from build123d import *

# Parameters (mm, degrees)
F1_DEPTH = 25.4
F2_W     = 50.8
F2_H     = 317.5
F3_DEPTH = 38.1
F4_W     = 50.8
F4_H     = 76.2
F5_DEPTH = 660.4
F7_DEPTH = 25.4
F8_W     = 1196.34
F8_H     = 25.4
F9_DEPTH = 304.8


# Not quite as in the source:
# - a feature names something its author has since deleted; it is built from what else it names


with BuildPart() as f1:
    # F0 (on Top) → F1 (new body)
    with BuildSketch(Plane.XY):
        Polygon((-674.37, -342.9), (674.37, -342.9), (674.37, 342.9), (-674.37, 342.9), (-674.37, -114.3), align=None)
    extrude(amount=F1_DEPTH)

    # F2 (on face) → F3 (join)
    with BuildSketch(Plane.XY.offset(25.4)):
        with Locations((-623.57, 44.45)):
            Rectangle(F2_W, F2_H)
        with Locations((623.57, 44.45)):
            Rectangle(F2_W, F2_H)
    extrude(amount=F3_DEPTH)

    # F4 (on face) → F5 (join)
    with BuildSketch(Plane.XY.offset(25.4)):
        with Locations((-623.57, -152.4)):
            Rectangle(F4_W, F4_H)
        with Locations((623.57, -152.4)):
            Rectangle(F4_W, F4_H)
    extrude(amount=F5_DEPTH)

    # F6 (on face) → F7 (join)
    with BuildSketch(Plane.XY.offset(685.8)):
        with BuildLine():
            ThreePointArc((-623.6857005119, -267.7317205817), (-605.7251882698, -260.2922328238), (-598.2857005119, -242.3317205817))
            Line((-598.2857005119, -242.3317205817), (-598.2857005119, 214.8682794183))
            ThreePointArc((-598.2857005119, 214.8682794183), (-605.7251882698, 232.8287916605), (-623.6857005119, 240.2682794183))
            ThreePointArc((-623.6857005119, 240.2682794183), (-641.6462127541, 232.8287916605), (-649.0857005119, 214.8682794183))
            Line((-649.0857005119, 214.8682794183), (-649.0857005119, -242.3317205817))
            ThreePointArc((-649.0857005119, -242.3317205817), (-641.6462127541, -260.2922328238), (-623.6857005119, -267.7317205817))
        make_face()
        with BuildLine():
            ThreePointArc((623.6857005119, -267.7317205817), (641.6462127541, -260.2922328238), (649.0857005119, -242.3317205817))
            Line((649.0857005119, -242.3317205817), (649.0857005119, 214.8682794183))
            ThreePointArc((649.0857005119, 214.8682794183), (641.6462127541, 232.8287916605), (623.6857005119, 240.2682794183))
            ThreePointArc((623.6857005119, 240.2682794183), (605.7251882698, 232.8287916605), (598.2857005119, 214.8682794183))
            Line((598.2857005119, 214.8682794183), (598.2857005119, -242.3317205817))
            ThreePointArc((598.2857005119, -242.3317205817), (605.7251882698, -260.2922328238), (623.6857005119, -267.7317205817))
        make_face()
    extrude(amount=F7_DEPTH)

    # F8 (on face) → F9 (join)
    with BuildSketch(Plane.XY.offset(25.4)):
        with Locations((0, -177.8)):
            Rectangle(F8_W, F8_H)
    extrude(amount=F9_DEPTH)


solid = f1.part
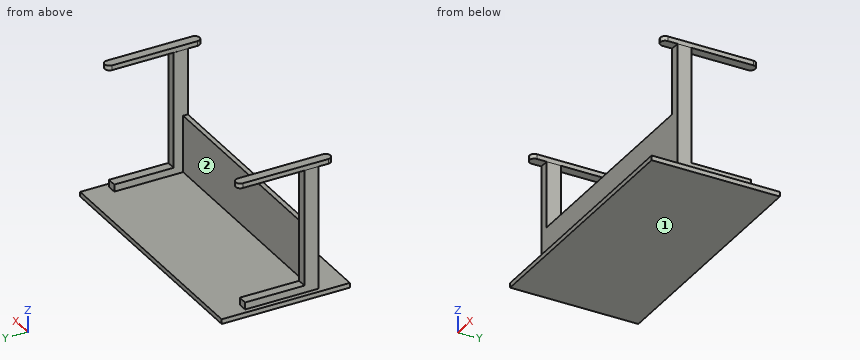
Check sheet for the modelled part. Datum: model origin and axes. Units: mm. Face numbers are marked on the shaded views. A direction names the side the tool comes from. Round coordinates to 2 decimals unless told otherwise and drop trailing zeros. Loops run counter-clockwise (first coordinate to the right, second up) from the corner with the lowest first, then second, coordinate; pieces in that order, holes last. Notation, with made-up numbers: (65, -14) - (112, -14) arc R20 ccw to (112, 17) - close; hole circle Ø1 at (59, 60). An arc over 180 degrees is marked (long way). Answer as CSV lines item,"result". Start each with the question number.
Item 1: Section check D-D (z = 133). Record the boundary of the cut face in (x, y), and give its area (3 significant figures).
Item 2: Section check C-C (x = -496). Record the boundary of the cut face in (y, z), and give its area (3 significant figures).
Item 3: Depth check by flat-ended pin: P1, Ø1.5, axis at x = -250, y = -213.5, coming from the -Z side; P2, Ø20.5, axis at x = 267, y = -177.5, coming from the +Z side; P3, Ø5, axis at x = 223.5, z = 209.5, coming from the +Y side; P4, Ø12.5, axis at y = -122.5, z = 699, coming from the -X side. Enter the tip coordinate at first touch or a pass-through.
Item 4: Scan lines: line 1 (X direction, y = -19.5, z = 34); line 2 (Z direction, x = 486.5, y = -305); line 3 (Y direction, x = 300.5, z = 137). Record each from-to range of solid material in increasing order. Write a range as [from, to].
Item 5: Section check A-A (z = 632.5). Record the boundary of the cut face in (x, y).
Item 6: Set-up check for the marked faces 1 and 2: record each of +Z, -Z, +X, -X, +Y, -Y from which the full face is reachable in a straight line by a thin tool's end or side.
Item 7: Section check B-B (y = 91). Record the boundary of the cut face in (x, z).
Report:
1,outline,"(-648.97, -190.5) - (648.97, -190.5) - (648.97, -114.3) - (598.17, -114.3) - (598.17, -165.1) - (-598.17, -165.1) - (-598.17, -114.3) - (-648.97, -114.3) - close"
1,area,"38,100 mm2"
2,outline,"(-342.9, 0) - (342.9, 0) - (342.9, 25.4) - (-165.1, 25.4) - (-165.1, 330.2) - (-190.5, 330.2) - (-190.5, 25.4) - (-342.9, 25.4) - close"
2,area,"25,200 mm2"
3,P1,"stops at z = 0"
3,P2,"stops at z = 330.2"
3,P3,"stops at y = -165.1"
3,P4,"stops at x = -649.09"
4,line 1,"x = [-648.97, -598.17], [598.17, 648.97]"
4,line 2,"z = [0, 25.4]"
4,line 3,"y = [-190.5, -165.1]"
5,outline,"(-648.97, -190.5) - (-598.17, -190.5) - (-598.17, -114.3) - (-648.97, -114.3) - close; (598.17, -190.5) - (648.97, -190.5) - (648.97, -114.3) - (598.17, -114.3) - close"
6,face 1,"-Z, +X, -X, +Y, -Y"
6,face 2,"+Z, +Y"
7,outline,"(-674.37, 0) - (674.37, 0) - (674.37, 25.4) - (648.97, 25.4) - (648.97, 63.5) - (598.17, 63.5) - (598.17, 25.4) - (-598.17, 25.4) - (-598.17, 63.5) - (-648.97, 63.5) - (-648.97, 25.4) - (-674.37, 25.4) - close; (-649.09, 685.8) - (-598.29, 685.8) - (-598.29, 711.2) - (-649.09, 711.2) - close; (598.29, 685.8) - (649.09, 685.8) - (649.09, 711.2) - (598.29, 711.2) - close"
